Source: CAD feature listing. Evaluate the final solid. Frame: model axes, mm. Round coordinates to 2 decimals unless told otherwise and drop trailing zeros. Write each loop counter-clockwise with the first axis right and the second up, starting at its lowest first coordinate (ties: lowest second). Pieces come first, ordered by that corner, then holes. Notation, with made-up numbers: M 65.25,-2.5 L 103.25,-2.5 A16 cw 103.25,15.5 Z; hole C 23.5,-27 d7. An arc over 180 degrees is marked long. Answer in a Markdown table with one row per item.
from build123d import *

# Parameters (mm, degrees)
SKETCH1_R           = 312.5
SKETCH1_R_2         = 156.25
BOSS_EXTRUDE1_DEPTH = 500
CHAMFER1_SIZE       = 12.5
FILLET1_R           = 50


with BuildPart() as part:
    # Sketch1 → Boss-Extrude1 (new body)
    with BuildSketch(Plane(origin=(0, 0, 0), x_dir=(0, 0, -1), z_dir=(1, 0, 0))):
        Circle(SKETCH1_R)
        Circle(SKETCH1_R_2, mode=Mode.SUBTRACT)
    extrude(amount=BOSS_EXTRUDE1_DEPTH)

    # Chamfer1
    chamfer1_edges = [part.edges().sort_by_distance(p)[0] for p in [
        (0, 0, 156.25),
        (500, 0, 156.25),
    ]]
    chamfer(chamfer1_edges, length=CHAMFER1_SIZE)

    # Fillet1
    fillet1_edges = [part.edges().sort_by_distance(p)[0] for p in [
        (0, 0, 312.5),
        (500, 0, 312.5),
    ]]
    fillet(fillet1_edges, radius=FILLET1_R)


solid = part.part
Q1. Section C-C (x = 273.5). Return loops of the section in (y, z).
Solutions:
| item | result |
|---|---|
| outline | C 0,0 d625; hole C 0,0 d312.5 |
Q2. Material intervals for probe 1 along Z at (x, y) = (189, -5.5); probe 2 along Y at (x, z) = (342, 0); probe 3 along Y at (x, z) = (438, -41.5), sorted ascending.
Solutions:
| item | result |
|---|---|
| probe 1 | z = -312.45 to -156.15, 156.15 to 312.45 |
| probe 2 | y = -312.5 to -156.25, 156.25 to 312.5 |
| probe 3 | y = -309.73 to -150.64, 150.64 to 309.73 |
Q3. Pull-direction query (Y, two-part tool) for faces 1 (the cylindrical face through (246.68, 154.92, 20.34)), 2 (the cylindrical face through (247.2, 309.84, 40.68)), 3 (the flat face through (500, -171, 4)); classes: pulls with the +Y half, pulls with the -Y half, needs draft (parallel to the pull), parting line crosses it, or undercut.
Solutions:
| item | result |
|---|---|
| face 1 | undercut |
| face 2 | parting line crosses it |
| face 3 | needs draft |
Q4. Section A-A (y = 0). Return loops of the section in (x, z), and give its area (3 significant figures).
Solutions:
| item | result |
|---|---|
| outline | M 0,-262.5 A50 ccw 50,-312.5 L 450,-312.5 A50 ccw 500,-262.5 L 500,-168.75 L 487.5,-156.25 L 12.5,-156.25 L 0,-168.75 Z; M 0,168.75 L 12.5,156.25 L 487.5,156.25 L 500,168.75 L 500,262.5 A50 ccw 450,312.5 L 50,312.5 A50 ccw 0,262.5 Z |
| area | 154,000 mm2 |
Q5. Contact query for flat-ended pins moving along their axis: pin 1 Ø4 at (y, z) = (87, 175) entering from -X; pin 2 Ø12 at (x, z) = (265.5, 197.5) entering from -Y; pin 3 Ø1 at (x, z) = (382.5, -249.5) entering from +Y; pin 4 Ø3 at (x, z) = (145.5, 83) entering from -Y. Output: stop coordinate, or through.
Solutions:
| item | result |
|---|---|
| pin 1 | stops at x = 0 |
| pin 2 | stops at y = -246.95 |
| pin 3 | stops at y = 188.83 |
| pin 4 | stops at y = -301.69 |
